Geometry: final body of the model. Coordinates: model frame, mm. Face numbers are marked on the shaded views. A direction names the side the tool comes from. Round coordinates to 2 decimals unless told otherwise and drop trailing zeros. Write each loop counter-clockwise with the first axis right and the second up, starting at its lowest first coordinate (ties: lowest second). Pieces come first, ordered by that corner, then holes. Notation, with made-up numbers: M -4,61 L 7,61 A8 cw 7,70 Z; hole C -14.5,80 d5. An arc over 180 degrees is marked long. Use one line per item in the form item = value. Start each with the question number.
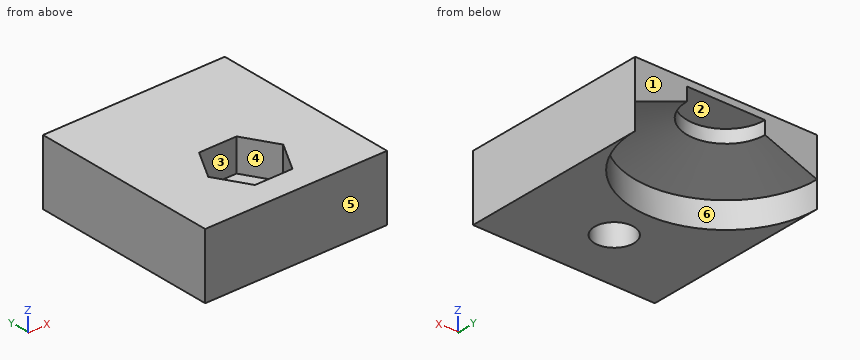
from build123d import *

# Parameters (mm, degrees)
REVOLUTION_ANGLE = -180
PAD011_DEPTH     = 10
POCKET002_DEPTH  = 5
SKETCH020_R      = 3
POCKET003_DEPTH  = 5


with BuildPart() as part:
    # Sketch017 → Revolution (revolve)
    with BuildSketch(Plane.XZ):
        Polygon((14, 0), (6, 3), (6, 5), (0, 5), (0, 6), (14, 6), align=None)
    revolve(axis=Axis((0, 0, 0), (0, 0, 1)), revolution_arc=REVOLUTION_ANGLE)

    # Sketch018 (on Face4 of Revolution) → Pad011 (new body)
    with BuildSketch(Plane(origin=(0, 0, 6), x_dir=(-1, 0, 0), z_dir=(0, 0, 1))):
        with BuildLine():
            Line((14, 0), (14, 29))
            Line((14, 29), (-14, 29))
            Line((-14, 29), (-14, 0))
            ThreePointArc((14, 0), (0, 14), (-14, 0))
        make_face()
    extrude(amount=-PAD011_DEPTH)

    # Sketch019 (on Face12 of Pad011) → Pocket002 (cut)
    with BuildSketch(Plane(origin=(0, 0, 6), x_dir=(-1, 0, 0), z_dir=(0, 0, 1))):
        Polygon((5.773503, 20), (2.886751, 25), (-2.886751, 25), (-5.773503, 20), (-2.886751, 15), (2.886751, 15), align=None)
    extrude(amount=-POCKET002_DEPTH, mode=Mode.SUBTRACT)

    # Sketch020 (on Face19 of Pocket002) → Pocket003 (cut)
    with BuildSketch(Plane(origin=(0, 0, 1), x_dir=(-1, 0, 0), z_dir=(0, 0, 1))):
        with Locations((0, 20)):
            Circle(SKETCH020_R)
    extrude(amount=-POCKET003_DEPTH, mode=Mode.SUBTRACT)


solid = part.part
1. Pull-direction query (Y, two-part tool) for the marked faces 1, 2 and 3; classes: released by +Y, released by -Y, zero draft, split by the parting line, or undercut.
2. Ray query, probe 1 along X at (y, z) = (-20, -2.5); probe 2 along Y at (x, z) = (0, -2.65); probe 3 along Z at (x, y) = (-4, -2.5). Return the intervals inside material, ascending.
3. Section query A-A (x = 0). Return loops of the section in (y, z), then the cut area to 3 significant figures.
4. Contact query for flat-ended pins moving along their axis: pin 1 (5 mm diameter, centred on x = 0, y = -20, fed in from +Z); pin 2 (3 mm diameter, centred on x = -1.5, y = -2.5, fed in from -Z); pin 3 (2 mm diameter, centred on x = -9.5, z = -1.5, fed in from +Y); pin 4 (3 mm diameter, centred on x = -1.5, y = -10.5, fed in from -Z). Output: stop coordinate, or through.
5. Section query C-C (z = 2.5). Return loops of the section in (x, y), then the cut area to 3 significant figures.
6. Section query B-B (z = -0.5). Return loops of the section in (x, y).
7. Set-up query: the marked faces 4, 5 and 6. Return all of +Z, -Z, +X, -X, +Y, -Y with unobstructed straight access to the full face (end or side cutting, diameter ignored); none if empty.
Checks:
q1.face_1 = released by +Y
q1.face_2 = zero draft
q1.face_3 = undercut
q2.probe_1 = -14 to -3, 3 to 14
q2.probe_2 = -29 to -23, -17 to -14
q2.probe_3 = 5 to 6
q3.outline = M -29,-4 L -23,-4 L -23,1 L -25,1 L -25,6 L -29,6 Z; M -17,-4 L -14,-4 L -14,0 L -6,3 L -6,5 L 0,5 L 0,6 L -15,6 L -15,1 L -17,1 Z
q3.area = 112 mm^2
q4.pin_1 = through
q4.pin_2 = 5
q4.pin_3 = -9.26
q4.pin_4 = 0.71
q5.outline = M -14,-29 L 14,-29 L 14,0 L 7.33,0 A7.33 cw -7.33,0 L -14,0 Z; hole M -5.77,-20 L -2.89,-25 L 2.89,-25 L 5.77,-20 L 2.89,-15 L -2.89,-15 Z
q5.area = 641 mm^2
q6.outline = M -14,-29 L 14,-29 L 14,0 A14 cw -14,0 Z; hole C 0,-20 d6
q7.face_4 = +Z
q7.face_5 = +Z, -Z, +X, -X, -Y
q7.face_6 = -Z, +Y
